Part model, mm, in its own coordinate system. A direction names the side the tool comes from. Give positions to 0.01 mm unless a question says otherwise; leave off trailing zeros. Write each loop counter-clockwise with the first axis right and the second up, starting at its lowest first coordinate (ties: lowest second). Pieces come first, ordered by that corner, then holes.
```python
from build123d import *

# Parameters (mm, degrees)
BOSS_EXTRUDE1_DEPTH   = 60
BOSS_EXTRUDE1_2_DEPTH = 60
SKETCH3_W             = 217
SKETCH3_H             = 10
BOSS_EXTRUDE3_DEPTH   = 20
SKETCH4_W             = 5
SKETCH4_H             = 70
BOSS_EXTRUDE4_DEPTH   = 50
SKETCH5_W             = 5
SKETCH5_H             = 70
BOSS_EXTRUDE5_DEPTH   = 50
SKETCH6_W             = 50
SKETCH6_H             = 45
CUT_EXTRUDE1_DEPTH    = 30
SKETCH7_W             = 50
SKETCH7_H             = 45
CUT_EXTRUDE2_DEPTH    = 20


with BuildPart() as part:
    # Sketch1 → Boss-Extrude1 (new body)
    with BuildSketch(Plane(origin=(0, 0, 0), x_dir=(1, 0, 0), z_dir=(0, 1, 0))):
        Polygon((0, 42.700803213), (0, 27.700803213), (0, 12.700803213), (94, -87.299196787), (94, 42.700803213), align=None)
        Polygon((79, -49.143729641), (79, 27.700803213), (17.378559694, 27.700803213), (17.378559694, 12.700803213), align=None, mode=Mode.SUBTRACT)
    extrude(amount=BOSS_EXTRUDE1_DEPTH)



with BuildPart() as body_2:
    # Sketch1 → Boss-Extrude1 2 (new body)
    with BuildSketch(Plane(origin=(0, 0, 0), x_dir=(1, 0, 0), z_dir=(0, 1, 0))):
        Polygon((-123, 12.700803213), (-123, -87.299196787), (-53, 12.700803213), (-53, 42.700803213), (-123, 42.700803213), align=None)
        Polygon((-108, 27.700803213), (-108, -39.713720468), (-68, 12.700803213), (-68, 27.700803213), align=None, mode=Mode.SUBTRACT)
    extrude(amount=BOSS_EXTRUDE1_2_DEPTH)

    # Sketch3 → Boss-Extrude3 (add)
    with BuildSketch(Plane(origin=(0, 60, 0), x_dir=(1, 0, 0), z_dir=(0, 1, 0))):
        with Locations((-14.5, 37.700803213)):
            Rectangle(SKETCH3_W, SKETCH3_H)
    extrude(amount=BOSS_EXTRUDE3_DEPTH)

    # Sketch4 → Boss-Extrude4 (add)
    with BuildSketch(Plane(origin=(0, 0, 0), x_dir=(-1, 0, 0), z_dir=(0, -1, 0))):
        with Locations((55.5, 77.700803213)):
            Rectangle(SKETCH4_W, SKETCH4_H)
    extrude(amount=-BOSS_EXTRUDE4_DEPTH)


with BuildPart() as part_1:
    add(part.part)

    add(body_2.part)  # Boss-Extrude5 merges body 2
    # Sketch5 → Boss-Extrude5 (add)
    with BuildSketch(Plane(origin=(0, 0, 0), x_dir=(-1, 0, 0), z_dir=(0, -1, 0))):
        with Locations((-2.5, 77.700803213)):
            Rectangle(SKETCH5_W, SKETCH5_H)
    extrude(amount=-BOSS_EXTRUDE5_DEPTH)

    # Sketch6 → Cut-Extrude1 (cut)
    with BuildSketch(Plane(origin=(94, 0, 0), x_dir=(0, 0, -1), z_dir=(1, 0, 0))):
        with Locations((-7.299196787, 29.5)):
            Rectangle(SKETCH6_W, SKETCH6_H)
    extrude(amount=-CUT_EXTRUDE1_DEPTH, mode=Mode.SUBTRACT)

    # Sketch7 → Cut-Extrude2 (cut)
    with BuildSketch(Plane.ZY.offset(123)):
        with Locations((7.299196787, 29.5)):
            Rectangle(SKETCH7_W, SKETCH7_H)
    extrude(amount=-CUT_EXTRUDE2_DEPTH, mode=Mode.SUBTRACT)


solid = part_1.part
```
1) 3-axis set-ups, long thin cutter, end or side, ignore diameter. For faces 4 (the face through (46.342, 29.58, 36.599)), 5 (the face through (-68, 30, -20)), 6 (the face through (-27, 60, -38)), 7 (the face through (-116, 29, 32.299)), 8 (the face through (87, 7, 8)): which of +Z, -Z, +X, -X, +Y, -Y reach the whole face in a straight line?
Answers follow:
face 4: +Z, +Y, -Y
face 5: +Y, -Y
face 6: +Z, -Z, -Y
face 7: -X
face 8: +X
2) Wall check: L1, parallel to X at y = 23, z = -27.5; L2, parallel to X at y = 10.5, z = -95.5; L3, parallel to Y at x = -74, z = 17. Give the ranges that are in metal, low to high.
Answers follow:
L1: x = -123 to -108, -68 to -53, 0 to 17.38, 79 to 94
L2: x = -58 to -53, 0 to 5
L3: y = 0 to 60
3) Saw through at B-B, the plane y = 14.5. Write the cut outline in (x, z).
Answers follow:
outline: (-123, -42.7) - (-58, -42.7) - (-58, -112.7) - (-53, -112.7) - (-53, -12.7) - (-123, 87.3) - (-123, 32.3) - (-108, 32.3) - (-108, 39.71) - (-68, -12.7) - (-68, -27.7) - (-108, -27.7) - (-108, -17.7) - (-123, -17.7) - close; (0, -112.7) - (5, -112.7) - (5, -42.7) - (94, -42.7) - (94, -17.7) - (79, -17.7) - (79, -27.7) - (17.38, -27.7) - (17.38, -12.7) - (79, 49.14) - (79, 32.3) - (94, 32.3) - (94, 87.3) - (0, -12.7) - close
4) Saw through at C-C, the plane x = -77. Write the cut outline in (y, z), then the cut area to 3 significant figures.
Answers follow:
outline: (0, -42.7) - (80, -42.7) - (80, -32.7) - (60, -32.7) - (60, -27.7) - (0, -27.7) - close; (0, -0.91) - (60, -0.91) - (60, 21.58) - (0, 21.58) - close
area: 2,450 mm2
5) Saw through at D-D, the plane z = -21. Write the cut outline in (x, y), then the cut area to 3 significant figures.
Answers follow:
outline: (-123, 0) - (-108, 0) - (-108, 60) - (-123, 60) - close; (-68, 0) - (-53, 0) - (-53, 60) - (-68, 60) - close; (0, 0) - (17.38, 0) - (17.38, 60) - (0, 60) - close; (79, 0) - (94, 0) - (94, 60) - (79, 60) - close
area: 3,740 mm2
6) Saw through at A-A, the plane z = -89.5. Write the cut outline in (x, y), then the cut area to 3 significant figures.
Answers follow:
outline: (-58, 0) - (-53, 0) - (-53, 50) - (-58, 50) - close; (0, 0) - (5, 0) - (5, 50) - (0, 50) - close
area: 500 mm2
7) Two-plate mould, pull along Y, no slides. Class faces 1 (the face through (-55, 50, -78)), 2 (the face through (-116, 52, 7)), 3 (the face through (51, 0, 24)): +Y half, -Y half, draft (parallel to the pull), parting line (faces both ways), or undercut.
Answers follow:
face 1: +Y half
face 2: undercut
face 3: -Y half
8) Pin check, flat tips, straight feed: pin 1 Ø8 at (x, y) = (-61.5, 62) entering from +Z; pin 2 Ø2.5 at (x, z) = (-56, -64) entering from +Y; pin 3 Ø18 at (y, z) = (33.5, -69) entering from +X; pin 4 Ø21 at (x, z) = (-72.5, 47) entering from +Y. Stop position of each tip, or through.
Answers follow:
pin 1: stops at z = 4.39
pin 2: stops at y = 50
pin 3: stops at x = 5
pin 4: passes through
